from build123d import *

# Parameters (mm, degrees)
SKETCH_W          = 75
SKETCH_H          = 12.7
PAD_DEPTH         = 12.7
SKETCH001_R       = 2
POCKET_DEPTH      = 6.351
POCKET_DEPTH_BACK = -6.351


with BuildPart() as part:
    # Sketch → Pad (new body)
    with BuildSketch(Plane.XY):
        Rectangle(SKETCH_W, SKETCH_H)
        with BuildLine():
            ThreePointArc((0, -4.898979), (8, 0), (0, 4.898979))
            ThreePointArc((0, 4.898979), (-8, 0), (0, -4.898979))
        make_face(mode=Mode.SUBTRACT)
    extrude(amount=PAD_DEPTH)

    # Sketch001 → Pocket (cut, two sides)
    with BuildSketch(Plane.XZ) as pocket_sk:
        with Locations((-32, 6.35)):
            Circle(SKETCH001_R)
        with Locations((-22, 6.35)):
            Circle(SKETCH001_R)
        with Locations((22, 6.35)):
            Circle(SKETCH001_R)
        with Locations((32, 6.35)):
            Circle(SKETCH001_R)
    extrude(amount=-POCKET_DEPTH, mode=Mode.SUBTRACT)
    extrude(pocket_sk.sketch, amount=-POCKET_DEPTH_BACK, mode=Mode.SUBTRACT)


solid = part.part
The listing builds one solid part. Answer for the finished solid, in the listing's coordinates (mm). Round coordinates to 2 decimals unless told otherwise and drop trailing zeros. Loops run counter-clockwise (first coordinate to the right, second up) from the corner with the lowest first, then second, coordinate; pieces in that order, holes last. Notation, with made-up numbers: M 48.5,55.5 L 59.5,55.5 A17 cw 59.5,70.5 Z; hole C -2,-20 d10. An arc over 180 degrees is marked long. Return JSON: item names as keys, results as strings.
Q1. Find section A-A, the plane x = -22. Determine the outline of the cut face in (y, z).
Results list:
{"outline": "M -6.35,0 L 6.35,0 L 6.35,4.35 L -6.35,4.35 Z; M -6.35,8.35 L 6.35,8.35 L 6.35,12.7 L -6.35,12.7 Z"}
Q2. Find section C-C, the plane z = 6.35. Determine the outline of the cut face in (x, y), plus the area to 3 significant figures.
Results list:
{"outline": "M -37.5,-6.35 L -34,-6.35 L -34,6.35 L -37.5,6.35 Z; M -30,-6.35 L -24,-6.35 L -24,6.35 L -30,6.35 Z; M -20,-6.35 L 20,-6.35 L 20,6.35 L -20,6.35 Z; M 24,-6.35 L 30,-6.35 L 30,6.35 L 24,6.35 Z; M 34,-6.35 L 37.5,-6.35 L 37.5,6.35 L 34,6.35 Z; hole M 0,-4.9 A5.5 ccw long 0,4.9 A5.5 ccw long Z", "area": "601 mm2"}
Q3. This flat-tipped pin is pushed along its axis until it touches: pin 1 Ø2.5 at (x, z) = (-32, 6.35) entering from +Y. Where does it stop, or does it pass through?
Results list:
{"pin 1": "passes through"}
Q4. Find section D-D, the plane x = 2.5. Determine the outline of the cut face in (y, z).
Results list:
{"outline": "M -6.35,0 L -5.5,0 L -5.5,12.7 L -6.35,12.7 Z; M 5.5,0 L 6.35,0 L 6.35,12.7 L 5.5,12.7 Z"}
Q5. Find the intervals of material crossed by line 1 along X through (y, z) = (-2, 5); line 2 along X through (y, z) = (0, 3.5); line 3 along Z through (x, y) = (-22, 3.75), in increasing order. Write a range as from..to.
Results list:
{"line 1": "x = -37.5..-33.48, -30.52..-23.48, -20.52..-7.62, 7.62..20.52, 23.48..30.52, 33.48..37.5", "line 2": "x = -37.5..-8, 8..37.5", "line 3": "z = 0..4.35, 8.35..12.7"}
Q6. The mould has two halves that part along X. Classify faces 1 (the face through (8, 0, 6)), 2 (the face through (37.5, 0, 6)), 3 (the face through (-1, 6, 0)): released by +X, released by -X, zero draft, split by the parting line, or undercut.
Results list:
{"face 1": "undercut", "face 2": "released by +X", "face 3": "zero draft"}
Q7. Find section B-B, the plane y = -1.5. Determine the outline of the cut face in (x, z), plus the area to 3 significant figures.
Results list:
{"outline": "M -37.5,0 L -7.79,0 L -7.79,12.7 L -37.5,12.7 Z; M 7.79,0 L 37.5,0 L 37.5,12.7 L 7.79,12.7 Z; hole C -32,6.35 d4; hole C -22,6.35 d4; hole C 22,6.35 d4; hole C 32,6.35 d4", "area": "704 mm2"}
